from build123d import *

# Parameters (mm, degrees)
SKETCH_OF_SERVO_MOTOR_W             = 42.5
SKETCH_OF_SERVO_MOTOR_H             = 54
EXTRUDE_BASE_OF_FOOT_DEPTH          = 5
POSITIONS_OF_FOOT_SIDES_W           = 5
POSITIONS_OF_FOOT_SIDES_H           = 54
POSITIONS_OF_FOOT_SIDES_H_2         = 6.8
EXTRUDE_SIDES_OF_FOOT_DEPTH         = 19
FILLET_TOP_EDGES_OF_SIDES_OF_FOOT_R = 3.5
EXTRUDE_FOOT_LIPS_DEPTH             = 42.5
FILLET_FOOT_LIPS_R                  = 4.1
HOLE_DIMENSIONS_FOR_M4_BOLT_R       = 2
EXTRUDE_CUT_HOLE_FOR_M4_BOLT_DEPTH  = 5


with BuildPart() as part:
    # Sketch of Servo Motor → Extrude Base of Foot (new body)
    with BuildSketch(Plane(origin=(0, 0, 0), x_dir=(1, 0, 0), z_dir=(0, 1, 0))):
        with Locations((10.65, -20.2)):
            Rectangle(SKETCH_OF_SERVO_MOTOR_W, SKETCH_OF_SERVO_MOTOR_H)
    extrude(amount=-EXTRUDE_BASE_OF_FOOT_DEPTH)

    # Positions of Foot Sides → Extrude Sides of Foot (add)
    with BuildSketch(Plane(origin=(0, 0, 0), x_dir=(1, 0, 0), z_dir=(0, 1, 0))):
        with Locations((29.4, -20.2)):
            Rectangle(POSITIONS_OF_FOOT_SIDES_W, POSITIONS_OF_FOOT_SIDES_H)
        with Locations((2.5, 3.4)):
            Rectangle(POSITIONS_OF_FOOT_SIDES_W, POSITIONS_OF_FOOT_SIDES_H_2)
        with Locations((2.5, -43.8)):
            Rectangle(POSITIONS_OF_FOOT_SIDES_W, POSITIONS_OF_FOOT_SIDES_H_2)
    extrude(amount=EXTRUDE_SIDES_OF_FOOT_DEPTH)

    # Fillet Top Edges of Sides of Foot
    fillet_top_edges_of_sides_of_foot_edges = [part.edges().sort_by_distance(p)[0] for p in [
        (2.5, 19, -6.8),
        (2.5, 19, 47.2),
        (29.4, 19, -6.8),
        (29.4, 19, 47.2),
    ]]
    fillet(fillet_top_edges_of_sides_of_foot_edges, radius=FILLET_TOP_EDGES_OF_SIDES_OF_FOOT_R)

    # Front and Back Foot Lips → Extrude Foot Lips (add, through all)
    with BuildSketch(Plane.ZY.offset(10.6)):
        Polygon((60.767406064, 4.5), (58.418174512, 7.855050358), (47.2, 0), (47.2, -5), align=None)
        Polygon((-6.8, 0), (-6.8, -5), (-20.367406064, 4.5), (-18.018174512, 7.855050358), align=None)
    extrude(amount=-EXTRUDE_FOOT_LIPS_DEPTH)

    # Fillet Foot Lips
    # the kernel refuses this fillet: 4.1 mm, written as the material it takes off along each edge
    with BuildSketch(Plane(origin=(-20.85, 4.5, 60.767406064), x_dir=(0, 0.8191520442889908, -0.5735764363510476), z_dir=(1, 0, 0)), Plane(origin=(-20.85, 4.5, -20.367406064), x_dir=(0, -0.5735764363510438, 0.8191520442889934), z_dir=(1, 0, 0))) as fillet_foot_lips_piece_1:
        with BuildLine():
            CenterArc((FILLET_FOOT_LIPS_R, -FILLET_FOOT_LIPS_R), FILLET_FOOT_LIPS_R, 90, 90)
            Line((0, -FILLET_FOOT_LIPS_R), (0, 0))
            Line((0, 0), (FILLET_FOOT_LIPS_R, 0))
        make_face()
    extrude(amount=63, mode=Mode.SUBTRACT)

    # Hole Dimensions for M4 Bolt → Extrude Cut Hole for M4 Bolt (cut)
    with BuildSketch(Plane.ZY):
        with Locations((-3.324953132, 14.258904835)):
            Circle(HOLE_DIMENSIONS_FOR_M4_BOLT_R)
        with Locations((-3.377058396, 4.358904835)):
            Circle(HOLE_DIMENSIONS_FOR_M4_BOLT_R)
        with Locations((43.724953132, 14.258904835)):
            Circle(HOLE_DIMENSIONS_FOR_M4_BOLT_R)
        with Locations((43.777058396, 4.358904835)):
            Circle(HOLE_DIMENSIONS_FOR_M4_BOLT_R)
    extrude(amount=-EXTRUDE_CUT_HOLE_FOR_M4_BOLT_DEPTH, mode=Mode.SUBTRACT)


solid = part.part
Here's how the part is built. I have some questions about the finished solid (model axes, mm). A direction names the side the tool comes from. Coordinates: 2 decimals unless noted, no trailing zeros. Order: outer loops, then holes, each group sorted by start corner. A loop starts at its lowest first (then second) coordinate and runs counter-clockwise, first axis right, second up. Notation, with made-up numbers: M 58,86.25 L 84,86.25 A13 ccw 84,97.25 Z; hole C -31,-12 d4. An arc over 180 degrees is marked long. Answer as CSV lines item,"result". Start each with the question number.
1. I need wall thicknesses on line 1 (Y direction, x = 26, z = 29.5); line 2 (Z direction, x = 29, y = 3.75); line 3 (Z direction, x = 18, y = 4.75). Which ranges of each line are inside material? Lowest first, please. Write a range as [from, to].
2. For pin 1 (4 mm diameter, centred on x = 22.5, y = 9, fed in from -Z); pin 2 (9.5 mm diameter, centred on y = 8, z = 33, fed in from -X); pin 3 (1.5 mm diameter, centred on x = 2, y = 11, fed in from -Z); pin 4 (5.5 mm diameter, centred on x = 28, y = 4, fed in from +Z), each with a flat end and sliding along its axis, tell me the tip position at first contact or that it passes through.
3. I want a section at D-D, the plane y = 17. Write out the boundary of the cut face in (x, z).
4. I want a section at B-B, the plane x = 26. Write out the boundary of the cut face in (y, z), and give its area (3 significant figures).
5. I want a section at C-C, the plane z = 36. Write out the boundary of the cut face in (x, y), and give its area (4 significant figures).
6. We'd pull the mould along Y, two halves only. Please class faces 6 (the cylindrical face through (2.465, 4.96, 45.685)), 7 (the flat face through (10.353, 3.983, 52.888)), 8 (the flat face through (0, 9, 44)): released by +Y, released by -Y, zero draft, split by the parting line, or undercut.
7. On a 3-axis mill with a long thin cutter (end or side, diameter ignored), from which of +Z, -Z, +X, -X, +Y, -Y can I reach the whole of each face in a straight line? I mean faces 1 (the cylindrical face through (2.465, 15.945, -2.25)), 2 (the flat face through (10.353, 3.983, -12.488)), 3 (the flat face through (26.9, 9, 21)), 4 (the flat face through (2, 9, 0)), 5 (the cylindrical face through (29.44, 18, 46.15)). Say none if no direction works.
8. I want a section at A-A, the plane y = 10.5. Write out the boundary of the cut face in (x, z).
Recorded:
1,line 1,"y = [-5, 0]"
1,line 2,"z = [-18.36, -12.16], [-6.8, 47.2], [52.56, 58.76]"
1,line 3,"z = [-18.69, -13.58], [53.98, 59.09]"
2,pin 1,"stops at z = -18.48"
2,pin 2,"stops at x = 26.9"
2,pin 3,"stops at z = -6.8"
2,pin 4,"stops at z = 59.16"
3,outline,"M 0,-6.46 L 5,-6.46 L 5,0 L 0,0 Z; M 0,40.4 L 5,40.4 L 5,46.86 L 0,46.86 Z; M 26.9,-6.46 L 31.9,-6.46 L 31.9,46.86 L 26.9,46.86 Z"
4,outline,"M -5,-6.8 L 2.15,-17.01 A4.1 ccw 7.86,-18.02 L 0,-6.8 L 0,47.2 L 7.86,58.42 A4.1 ccw 2.15,57.41 L -5,47.2 Z"
4,area,"387 mm2"
5,outline,"M -10.6,-5 L 31.9,-5 L 31.9,19 L 26.9,19 L 26.9,0 L -10.6,0 Z"
5,area,"307.5 mm2"
6,face 6,"undercut"
6,face 7,"released by +Y"
6,face 8,"zero draft"
7,face 1,"-X"
7,face 2,"+X, -X, +Y"
7,face 3,"+Y"
7,face 4,"-X, +Y"
7,face 5,"+Z, +X, -X, +Y"
8,outline,"M 0,-6.8 L 5,-6.8 L 5,0 L 0,0 Z; M 0,40.4 L 5,40.4 L 5,47.2 L 0,47.2 Z; M 26.9,-6.8 L 31.9,-6.8 L 31.9,47.2 L 26.9,47.2 Z"
